Source: CAD feature listing. Evaluate the final solid. Frame: model axes, mm. Round coordinates to 2 decimals unless told otherwise and drop trailing zeros. Loops run counter-clockwise (first coordinate to the right, second up) from the corner with the lowest first, then second, coordinate; pieces in that order, holes last. Notation, with made-up numbers: (89, -26) - (113, -26) arc R28 cw to (113, 2) - close; hole circle Ø8 at (-4.5, -39.5). An arc over 180 degrees is marked (long way). One line per question, with ' | ' between items.
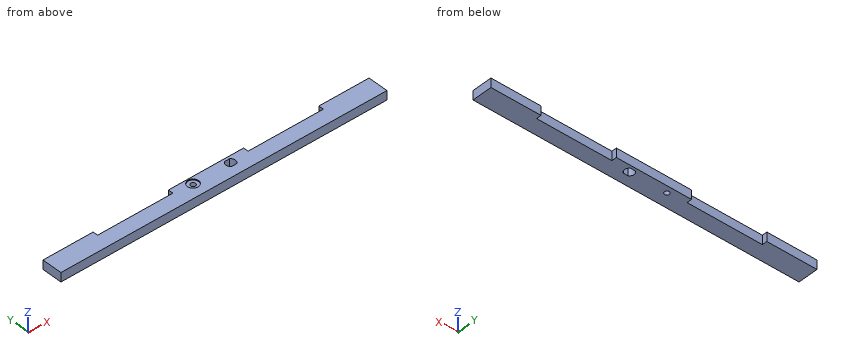
from build123d import *

# Parameters (mm, degrees)
PAD_DEPTH          = 18
SKETCH001_R        = 11
SKETCH001_R_2      = 4.9
POCKET_DEPTH       = 2
POCKET001_DEPTH    = 20
POCKET001_FACE30_R = 4.9
POCKET002_DEPTH    = 20


with BuildPart() as part:
    # Sketch → Pad (new body)
    with BuildSketch(Plane.XY):
        Polygon((0, 0), (-325, 0), (-325, 40), (-225, 40), (-225, 30), (-75, 30), (-75, 40), (0, 40), align=None)
    pad = extrude(amount=PAD_DEPTH)

    # Mirrored: Pad across Sketch V_Axis
    add(pad.mirror(Plane(origin=(0, 0, 0), x_dir=(0, 0, 1), z_dir=(1, 0, 0))))

    # Sketch001 (on DatumPlane) → Pocket (cut)
    with BuildSketch(Plane.XY.offset(18)):
        with Locations((-37.5, 27)):
            Circle(SKETCH001_R)
        with Locations((-37.5, 27)):
            Circle(SKETCH001_R_2, mode=Mode.SUBTRACT)
        with BuildLine():
            ThreePointArc((32.592862, 34.9), (28.2, 27), (32.592862, 19.1))
            Line((32.592862, 19.1), (42.407138, 19.1))
            ThreePointArc((42.407138, 19.1), (46.8, 27), (42.407138, 34.9))
            Line((32.592862, 34.9), (42.407138, 34.9))
        make_face()
    extrude(amount=-POCKET_DEPTH, mode=Mode.SUBTRACT)

    # Pocket Face25 → Pocket001 (cut)
    with BuildSketch(Plane(origin=(37.5, 27, 16), x_dir=(0, 1, 0), z_dir=(0, 0, 1))):
        with BuildLine():
            ThreePointArc((7.9, 4.907138), (0, 9.3), (-7.9, 4.907138))
            Line((-7.9, 4.907138), (-7.9, -4.907138))
            ThreePointArc((-7.9, -4.907138), (0, -9.3), (7.9, -4.907138))
            Line((7.9, -4.907138), (7.9, 4.907138))
        make_face()
    extrude(amount=-POCKET001_DEPTH, mode=Mode.SUBTRACT)

    # Pocket001 Face30 → Pocket002 (cut)
    with BuildSketch(Plane(origin=(-37.5, 27, 18), x_dir=(0, 1, 0), z_dir=(0, 0, 1))):
        Circle(POCKET001_FACE30_R)
    extrude(amount=-POCKET002_DEPTH, mode=Mode.SUBTRACT)


solid = part.part
1. Material intervals for probe 1 along X at (y, z) = (38, 12.75); probe 2 along Y at (x, z) = (-37.5, 16.9); probe 3 along X at (y, z) = (29, 15), sorted ascending.
Worked out:
probe 1: x = -325 to -225, -75 to 75, 225 to 325 | probe 2: y = 0 to 16, 38 to 40 | probe 3: x = -325 to -41.97, -33.03 to 28.42, 46.58 to 325
2. Section query B-B, the plane x = -161. Return loops of the section in (y, z).
Worked out:
outline: (0, 0) - (30, 0) - (30, 18) - (0, 18) - close
3. Contact query for flat-ended pins moving along their axis: P1, Ø5, axis at x = 139.5, z = 10.5, coming from the +Y side; P2, Ø11.5, axis at x = -37.5, y = 27, coming from the +Z side. Output: stop coordinate, or through.
Worked out:
P1: stops at y = 30 | P2: stops at z = 16
4. Section query A-A, the plane z = 5.5. Return loops of the section in (x, y), plus the area to 3 significant figures.
Worked out:
outline: (-325, 0) - (325, 0) - (325, 40) - (225, 40) - (225, 30) - (75, 30) - (75, 40) - (-75, 40) - (-75, 30) - (-225, 30) - (-225, 40) - (-325, 40) - close; hole circle Ø9.8 at (-37.5, 27); hole (32.59, 19.1) - (42.41, 19.1) arc R9.3 ccw to (42.41, 34.9) - (32.59, 34.9) arc R9.3 ccw to start | area: 22,700 mm2
